CAD build for the part. Positions are in the model's coordinates, mm. A direction names the side the tool comes from. Coordinates: 2 decimals unless noted, no trailing zeros. Write each loop counter-clockwise with the first axis right and the second up, starting at its lowest first coordinate (ties: lowest second). Pieces come first, ordered by that corner, then holes.
```python
from build123d import *

# Parameters (mm, degrees)
F2_R      = 25
F3_DEPTH  = 1.5
F4_R      = 16
F5_DEPTH  = 12
F6_R      = 20.5
F7_DEPTH  = 3
F8_R      = 16
F9_DEPTH  = 8
F10_R     = 6
F11_DEPTH = 63.501


with BuildPart() as f1:
    # F0 (on Front) → F1 (revolve)
    with BuildSketch(Plane.XZ):
        with BuildLine():
            Line((0, 25), (0, 0))
            Line((0, 0), (88, 0))
            Line((88, 0), (88, 16))
            Line((88, 16), (85, 16))
            Line((85, 16), (85, 20))
            Line((85, 20), (68, 20))
            Line((68, 20), (68, 31))
            Line((68, 31), (56, 31))
            ThreePointArc((56, 31), (50, 25), (44, 31))
            Line((44, 31), (6, 31))
            ThreePointArc((6, 31), (1.7573593129, 29.2426406871), (0, 25))
        make_face()
    revolve(axis=Axis((44, 0, 0), (1, 0, 0)))

    # F2 (on face) → F3 (cut)
    with BuildSketch(Plane(origin=(0, 0, 0), x_dir=(0, -1, 0), z_dir=(-1, 0, 0))):
        Circle(F2_R)
    extrude(amount=-F3_DEPTH, mode=Mode.SUBTRACT)

    # F4 (on face) → F5 (cut)
    with BuildSketch(Plane(origin=(1.5, 0, 0), x_dir=(0, -1, 0), z_dir=(-1, 0, 0))):
        Circle(F4_R)
    extrude(amount=-F5_DEPTH, mode=Mode.SUBTRACT)

    # F6 (on face) → F7 (cut)
    with BuildSketch(Plane(origin=(13.5, 0, 0), x_dir=(0, -1, 0), z_dir=(-1, 0, 0))):
        Circle(F6_R)
    extrude(amount=-F7_DEPTH, mode=Mode.SUBTRACT)

    # F8 (on face) → F9 (cut)
    with BuildSketch(Plane(origin=(16.5, 0, 0), x_dir=(0, -1, 0), z_dir=(-1, 0, 0))):
        Circle(F8_R)
    extrude(amount=-F9_DEPTH, mode=Mode.SUBTRACT)

    # F10 (on face) → F11 (cut, through all)
    with BuildSketch(Plane(origin=(24.5, 0, 0), x_dir=(0, -1, 0), z_dir=(-1, 0, 0))):
        Circle(F10_R)
    extrude(amount=-F11_DEPTH, mode=Mode.SUBTRACT)


solid = f1.part
```
Item 1: Wall check: line 1 along Z through (x, y) = (9.25, 0); line 2 along Z through (x, y) = (15.45, 0); line 3 along X through (y, z) = (18, -1). Give the ranges that are in metal, low to high.
Item 2: Flat gauge pins, fed straight in: pin 1 Ø15.5 at (y, z) = (0, 0) entering from -X; pin 2 Ø2 at (x, y) = (30, 17.5) entering from +Z; pin 3 Ø20.5 at (y, z) = (-4.5, -5) entering from -X. Where does each tip first touch, or does it go through?
Item 3: Saw through at B-B, the plane x = 60. Write the cut outline in (y, z).
Item 4: Saw through at A-A, the plane x = 76.5. Write the cut outline in (y, z), and give its area (3 significant figures).
Item 5: Which spindle directions (+Z, -Z, +X, -X, +Y, -Y) get a long thin tool onto all of the face, cutting with end or side? Do faces 1 (the cylindrical face through (14.979, 4.444, -20.013)), 2 (the flat face through (24.5, -7, 0)), 3 (the cylindrical face through (76.381, 19.524, -4.336)). Say none if no direction does.
Item 6: Two-plate mould, pull along X, no slides. Class faces 4 (the flat face through (88, 0, -7)), 5 (the flat face through (13.5, -12, -11)), 6 (the cylindrical face through (24.734, -30.736, -4.036)): +X half, -X half, draft (parallel to the pull), parting line (faces both ways), or undercut.
Working result:
1. line 1: z = -31 to -16, 16 to 31
1. line 2: z = -31 to -20.5, 20.5 to 31
1. line 3: x = 1.5 to 13.5, 16.5 to 85
2. pin 1: stops at x = 24.5
2. pin 2: stops at z = 26.24
2. pin 3: stops at x = 1.5
3. outline: circle Ø62 at (0, 0); hole circle Ø12 at (0, 0)
4. outline: circle Ø40 at (0, 0); hole circle Ø12 at (0, 0)
4. area: 1,140 mm2
5. face 1: none
5. face 2: -X
5. face 3: +X
6. face 4: +X half
6. face 5: undercut
6. face 6: draft
